from build123d import *

# Parameters (mm, degrees)
F0_W           = 200
F0_H           = 180
F0_W_2         = 9
F0_H_2         = 75
F0_W_3         = 120
F0_H_3         = 41
F0_W_4         = 71
F0_H_4         = 25
F0_W_5         = 31
F0_H_5         = 15
F1_DEPTH       = 3
F4_D           = 8.8
F4_CSINK_D     = 20
F4_CSINK_ANGLE = 90
F5_D           = 25
F6_D           = 25


# Not quite as in the source:
# - a feature of the source that left no trace in its solid (it failed there, or was rolled back) is left out
# - the program builds the solid bodies; features that only make, move or delete a surface that nothing else refers to are left out


with BuildPart() as f1:
    # F0 (on Top) → F1 (new body)
    with BuildSketch(Plane.XY):
        with Locations((0.7408946753, -7.6781137288)):
            Rectangle(F0_W, F0_H)
        with Locations((4.5, -57.5837731361)):
            Rectangle(F0_W_2, F0_H_2, mode=Mode.SUBTRACT)
        with Locations((-30.8628822118, 55.5105576217)):
            Rectangle(F0_W_3, F0_H_3, mode=Mode.SUBTRACT)
        with Locations((21.3823994361, 13.5011318373)):
            Rectangle(F0_W_4, F0_H_4, mode=Mode.SUBTRACT)
        with Locations((58.7239102691, 41.1898118258)):
            Rectangle(F0_W_5, F0_H_5, mode=Mode.SUBTRACT)
        with Locations((58.7239102691, 64.3030141294)):
            Rectangle(F0_W_5, F0_H_5, mode=Mode.SUBTRACT)
    extrude(amount=F1_DEPTH)

    # F4 (through all)
    with Locations(Plane.XY.offset(3)):
        with Locations((-51.7591053247, -55.4611310363)):
            CounterSinkHole(F4_D / 2, F4_CSINK_D / 2, counter_sink_angle=F4_CSINK_ANGLE)

    # F5 (through all)
    with Locations(Plane.XY.offset(3)):
        with Locations((65.8319948756, -54.5700079396)):
            Hole(F5_D / 2)

    # F6 (through all)
    with Locations(Plane.XY.offset(3)):
        with Locations((-62.68462408, 6.748889561)):
            Hole(F6_D / 2)


solid = f1.part
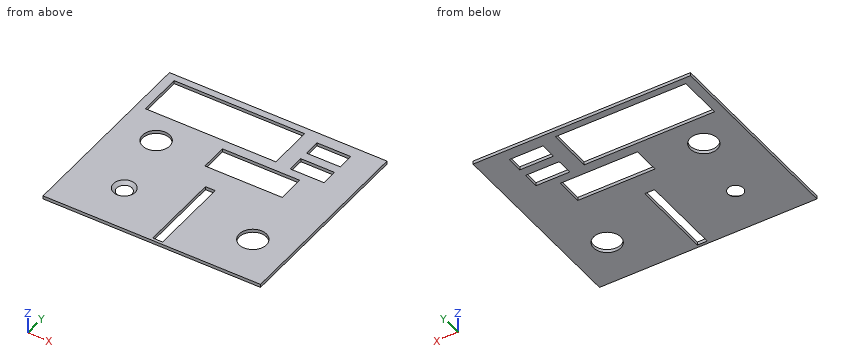
Input: part model. Units: mm. Frame: model coordinates. Give positions to 0.01 mm unless a question says otherwise; leave off trailing zeros. Write each loop counter-clockwise with the first axis right and the second up, starting at its lowest first coordinate (ties: lowest second). Pieces come first, ordered by that corner, then holes. Notation, with made-up numbers: M -25,75 L -3,75 A29 cw -3,105 Z; hole C 10,-29.5 d2. An arc over 180 degrees is marked long. Write item = value, one per line. Start each with the question number.
1) First-contact query: pin 1 Ø12 at (x, y) = (-62, 8) entering from -Z. Flat tip, straight axial feed; report the tip coordinate or a pass-through.
2) Cut plane D-D on y = -38. Return the cut outline in (x, z).
3) Cut plane A-A on x = -11. Return the cut outline in (y, z), then the cut area to 3 significant figures.
4) Material intervals for line 1 along Y through (x, z) = (16, 1.35); line 2 along X through (y, z) = (39.5, 1.95); line 3 along Y through (x, z) = (49, 0.9), sorted ascending. Write a range as [from, to].
5) Cut plane B-B on y = 39.5. Return the cut outline in (x, z).
6) Cut plane C-C on z = 0.95. Count the separate pieces of the cut face and the enclosed holes in it, then the cut area to 3 significant figures.
Solved:
q1.pin_1 = through
q2.outline = M -99.26,0 L 0,0 L 0,3 L -99.26,3 Z; M 9,0 L 100.74,0 L 100.74,3 L 9,3 Z
q3.outline = M -97.68,0 L 1,0 L 1,3 L -97.68,3 Z; M 26,0 L 35.01,0 L 35.01,3 L 26,3 Z; M 76.01,0 L 82.32,0 L 82.32,3 L 76.01,3 Z
q3.area = 342 mm2
q4.line_1 = [-97.68, 1], [26, 35.01], [76.01, 82.32]
q4.line_2 = [-99.26, -90.86], [29.14, 43.22], [74.22, 100.74]
q4.line_3 = [-97.68, 1], [26, 33.69], [48.69, 56.8], [71.8, 82.32]
q5.outline = M -99.26,0 L -90.86,0 L -90.86,3 L -99.26,3 Z; M 29.14,0 L 43.22,0 L 43.22,3 L 29.14,3 Z; M 74.22,0 L 100.74,0 L 100.74,3 L 74.22,3 Z
q6.separate_pieces = 1
q6.enclosed_holes = 8
q6.area = 26,500 mm2
